Autodesk Inventor part; units mm, degrees
ref_plane "YZ Plane" through (0, 0, 0) normal (1, 0, 0) x (0, 1, 0)
ref_plane "XZ Plane" through (0, 0, 0) normal (0, 1, 0) x (-1, 0, 0)
ref_plane "XY Plane" through (0, 0, 0) normal (0, 0, 1) x (1, 0, 0)
sketch "Sketch1" plane through (0, 0, 0) normal (0, 1, 0) x (-1, 0, 0)
  line L0 (-27.5, 6) -> (-15, 6)
  line L1 (-15, 6) -> (-18, 0)
  line L2 (-27.5, 25) -> (-27.5, 6)
  line L3 (-27.5, 25) -> (0, 25)
  line L4 (-18, 0) -> (0, 0)
  line L5 (0, -5) -> (0, 30)
  line L6 (38.5, 0) -> (-38.5, 0)
  line L7 (27.5, 6) -> (15, 6)
  line L8 (15, 6) -> (18, 0)
  line L9 (27.5, 25) -> (27.5, 6)
  line L10 (27.5, 25) -> (0, 25)
  line L11 (18, 0) -> (0, 0)
  dimension "d9" = 19
  dimension "d10" = 25
  dimension "d11" = 27.5
  dimension "d17" = 12.5
  dimension "d19" = 9.5
extrude "Extrusion1" add sketch "Sketch1" along normal mid plane 20
sketch "Sketch2" plane through (0, -10, 0) normal (0, -1, 0) x (1, 0, 0)
  line L0 (18, 0) -> (-18, 0)
  line L1 (-27.5, 25) -> (27.5, 25)
  point P0 (0, 0)
  point P1 (0, 15)
  point P2 (0, 0)
  dimension "d20" = 10
hole "Hole1" at (0, -10, 15) direction (0, 1, 0) diameter 12 depth 10
sketch "Sketch3" plane through (-27.5, 10, 25) normal (0, 0, 1) x (1, 0, 0)
  line L0 (19.5, -16) -> (35.5, -16)
  line L1 (37.5, -14) -> (37.5, -6)
  line L2 (35.5, -4) -> (19.5, -4)
  line L3 (17.5, -6) -> (17.5, -14)
  arc A0 (17.5, -14) -> (19.5, -16) centre (19.5, -14) ccw
  arc A1 (35.5, -16) -> (37.5, -14) centre (35.5, -14) ccw
  arc A2 (37.5, -6) -> (35.5, -4) centre (35.5, -6) ccw
  arc A3 (19.5, -4) -> (17.5, -6) centre (19.5, -6) ccw
  line L4 (-11, -10) -> (66, -10) construction
  line L5 (27.5, 4) -> (27.5, -24) construction
  point P0 (27.5, -10)
  point P1 (27.5, -4)
  point P2 (17.5, -10)
  dimension "d28" = 2
  dimension "d29" = 20
  dimension "d30" = 12
extrude "Extrusion2" cut sketch "Sketch3" against normal blind 16
sketch "Sketch4" plane through (0, 10, 0) normal (0, 1, 0) x (1, 0, 0)
  line L0 (27.5, -25) -> (-27.5, -25)
  line L1 (27.5, -6) -> (27.5, -25)
  line L2 (-27.5, -25) -> (-27.5, -6)
  point P0 (0, 0)
  point P1 (-17.5, -16)
  point P2 (17.5, -16)
  dimension "d37" = 10
  dimension "d38" = 9
  dimension "d39" = 10
hole "Hole2" at (-17.5, 10, 16) at (17.5, 10, 16) direction (0, -1, 0) diameter 4.134 depth 8 tip angle 118
chamfer "Chamfer1" distance 3 angle 45 2 edges at (27.5, 0, 25) (-27.5, 0, 25)
equation "\"d3\" = 0.5"
equation "\"d4\" = 25"
properties part number "Slider"
Input: part model. Units: mm. Frame: model coordinates. A direction names the side the tool comes from. Give positions to 0.01 mm unless a question says otherwise; leave off trailing zeros. Order: outer loops, then holes, each group sorted by start corner. A loop starts at its lowest first (then second) coordinate and runs counter-clockwise, first axis right, second up. Notation, with made-up numbers: (26, -27.5) -> (66, -27.5) arc R30 cw to (66, 5.5) -> close; hole circle Ø5 at (58, 81). An arc over 180 degrees is marked (long way). Write each question's results on one line, items separated by ' | '. Start each with the question number.
Item 1: Set-up query: faces 4 (the flat face through (21, 0, 6)), 5 (the cylindrical face through (2.3, -7.97, 9.46)), 6 (the cylindrical face through (9.4, -5.43, 17.11)). Return all of +Z, -Z, +X, -X, +Y, -Y with unobstructed straight access to the full face (end or side cutting, diameter ignored); none if empty.
Item 2: Cut plane D-D on y = 5. Return the cut outline in (x, z).
Item 3: Cut plane C-C on x = 7. Return the cut outline in (y, z).
Item 4: Cut plane B-B on y = -2. Return the cut outline in (x, z), then the cut area to 3 significant figures.
Item 5: Mould query, pull axis Y, two halves, no side actions, for faces 1 (the flat face through (0, 10, 13)), 2 (the cylindrical face through (15.757, 5.944, 17.111)), 3 (the flat face through (10, 0, 17)). Classes: pulls with the +Y half, pulls with the -Y half, needs draft (parallel to the pull), parting line crosses it, or undercut.
Item 6: Contact query for a flat-ended pin moving along its axis: P1, Ø1, axis at y = -6.5, z = 3.5, coming from the -X side. Output: stop coordinate, or through.
Item 7: Line query: line 1 (X direction, y = 7.5, z = 16); line 2 (X direction, y = -9.1, z = 15); line 3 (Z direction, x = 17.5, y = 7). Output: solid intervals per line, ascending.
Item 8: Cut plane A-A on y = -7. Return the cut outline in (x, z), then the cut area to 3 significant figures.
Established:
1) face 4: +X, +Y, -Y | face 5: -Y | face 6: +Z
2) outline: (-27.5, 6) -> (-15, 6) -> (-18, 0) -> (18, 0) -> (15, 6) -> (27.5, 6) -> (27.5, 22) -> (24.5, 25) -> (9.73, 25) -> (9.73, 9) -> (-9.73, 9) -> (-9.73, 25) -> (-24.5, 25) -> (-27.5, 22) -> close; hole circle Ø4.13 at (-17.5, 16); hole circle Ø4.13 at (17.5, 16)
3) outline: (-10, 0) -> (10, 0) -> (10, 25) -> (6, 25) -> (6, 9) -> (-6, 9) -> (-6, 25) -> (-10, 25) -> close
4) outline: (-27.5, 6) -> (-15, 6) -> (-18, 0) -> (18, 0) -> (15, 6) -> (27.5, 6) -> (27.5, 22) -> (24.5, 25) -> (10, 25) -> (10, 9) -> (-10, 9) -> (-10, 25) -> (-24.5, 25) -> (-27.5, 22) -> close | area: 914 mm^2
5) face 1: pulls with the +Y half | face 2: needs draft | face 3: undercut
6) P1: x = -16.5
7) line 1: -27.5 to -19.57, -15.43 to 15.43, 19.57 to 27.5 | line 2: -27.5 to -6, 6 to 27.5 | line 3: 0 to 1, 6 to 13.93, 18.07 to 25
8) outline: (-27.5, 6) -> (-15, 6) -> (-18, 0) -> (18, 0) -> (15, 6) -> (27.5, 6) -> (27.5, 22) -> (24.5, 25) -> (-24.5, 25) -> (-27.5, 22) -> close; hole circle Ø12 at (0, 15) | area: 1,120 mm^2
